The listing builds one solid part. Answer for the finished solid, in the listing's coordinates (mm). A direction names the side the tool comes from. Coordinates: 2 decimals unless noted, no trailing zeros. Order: outer loops, then holes, each group sorted by start corner. A loop starts at its lowest first (then second) coordinate and runs counter-clockwise, first axis right, second up. Notation, with made-up numbers: (12, -11) - (29, -11) arc R22 ccw to (29, 0) - close; hole circle Ø10 at (3, 50.5). An arc over 180 degrees is marked (long way). Use a Markdown table: item, result. Add a question column.
Item 1: Find the intervals of material crossed by line 1 along Z through (x, y) = (78.5, 0); line 2 along X through (y, z) = (3, 3.75); line 3 along X through (y, z) = (1.25, -3.5), in increasing order.
Item 2: The mould has two halves that part along X. Classify faces 6 (the cylindrical face through (129, -0.1, -2.9)), 7 (the flat face through (5.5, 0, -2)), 8 (the cylindrical face through (3.22, -3.75, 0.02)): released by +X, released by -X, zero draft, split by the parting line, or undercut.
Item 3: Flat-ended cylindrical pins translate along their axes: P1, Ø1, axis at x = 24.5, z = 0, coming from the -Y side; P2, Ø0.6, axis at x = 120, y = 0, coming from the +Z side; P3, Ø0.8, axis at x = 122, z = 2.5, coming from the -Y side; P4, Ø3, axis at y = -0.5, z = 0, coming from the -X side. Find the tip coordinate at first contact, or state that the pin passes through.
Item 4: The part is cut by section B-B, the plane x = 17. Give the vertices of the cut face in (y, z), then the cut area to 3 significant figures.
Item 5: For faces 1 (the flat face through (7, -4, -1)), 2 (the flat face through (3, 0, -1.25)), 3 (the flat face through (3, 0, 1.25)), 4 (the flat face through (122, 0, 1.8)), 5 (the cylindrical face through (3.22, 3.75, -0.02)), determine the directions among +Z, -Z, +X, -X, +Y, -Y from which every point of the face is accessible in a straight line to the end or side of a thin tool.
Item 6: The part is cut by section A-A, the plane z = 0. Give the vertices of the cut face in (x, y), then the cut area to 3 significant figures.
from build123d import *

# Parameters (mm, degrees)
F2_SIZE  = 1
F4_DEPTH = 5.5
F7_DEPTH = 1.2


with BuildPart() as f1:
    # F0 (on Front) → F1 (revolve)
    with BuildSketch(Plane.XZ):
        Polygon((0, 3.75), (0, 0), (130, 0), (130, 3), (129.3, 3), (129.3, 2.9), (128.7, 2.9), (128.7, 3), (115, 3), (115, 3.75), (7, 3.75), (7, 5), (5.5, 5), (5.5, 3.75), align=None)
    revolve(axis=Axis((81.1427264533, 0, 0), (1, 0, 0)))

    # F2
    f2_edges = [f1.edges().sort_by_distance(p)[0] for p in [
        (0, 0, -3.75),
    ]]
    chamfer(f2_edges, length=F2_SIZE)

    # F3 (on face) → F4 (cut, through all)
    with BuildSketch(Plane(origin=(0, 0, 0), x_dir=(0, -1, 0), z_dir=(-1, 0, 0))):
        with BuildLine():
            Line((2.4494897428, 1.25), (3.5355339059, 1.25))
            ThreePointArc((3.5355339059, 1.25), (0, 3.75), (-3.5355339059, 1.25))
            Line((-3.5355339059, 1.25), (-2.4494897428, 1.25))
            ThreePointArc((-2.4494897428, 1.25), (0, 2.75), (2.4494897428, 1.25))
        make_face()
        with BuildLine():
            ThreePointArc((-3.5355339059, -1.25), (0, -3.75), (3.5355339059, -1.25))
            Line((3.5355339059, -1.25), (2.4494897428, -1.25))
            ThreePointArc((2.4494897428, -1.25), (0, -2.75), (-2.4494897428, -1.25))
            Line((-2.4494897428, -1.25), (-3.5355339059, -1.25))
        make_face()
        with BuildLine():
            Line((-2.4494897428, 1.25), (2.4494897428, 1.25))
            ThreePointArc((2.4494897428, 1.25), (0, 2.75), (-2.4494897428, 1.25))
        make_face()
        with BuildLine():
            ThreePointArc((-2.4494897428, -1.25), (0, -2.75), (2.4494897428, -1.25))
            Line((2.4494897428, -1.25), (-2.4494897428, -1.25))
        make_face()
    extrude(amount=-F4_DEPTH, mode=Mode.SUBTRACT)

    # F6 (on offset) → F7 (cut, through all)
    with BuildSketch(Plane.XY.offset(1.8)):
        with BuildLine():
            ThreePointArc((125, -1), (126, 0), (125, 1))
            Line((125, 1), (119, 1))
            ThreePointArc((119, 1), (118, 0), (119, -1))
            Line((119, -1), (125, -1))
        make_face()
    extrude(amount=F7_DEPTH, mode=Mode.SUBTRACT)


solid = f1.part
Solution:
| question | item | result |
|---|---|---|
| 1 | line 1 | z = -3.75 to 3.75 |
| 1 | line 2 | x = 5.5 to 7 |
| 1 | line 3 | x = 5.5 to 115 |
| 2 | face 6 | undercut |
| 2 | face 7 | released by -X |
| 2 | face 8 | zero draft |
| 3 | P1 | stops at y = -3.75 |
| 3 | P2 | stops at z = 1.8 |
| 3 | P3 | stops at y = -2.14 |
| 3 | P4 | stops at x = 0 |
| 4 | outline | circle Ø7.5 at (0, 0) |
| 4 | area | 44.2 mm2 |
| 5 | face 1 | +X |
| 5 | face 2 | -Z, -X, +Y, -Y |
| 5 | face 3 | +Z, -X, +Y, -Y |
| 5 | face 4 | +Z |
| 5 | face 5 | -X, +Y |
| 6 | outline | (0, -2.75) - (1, -3.75) - (5.5, -3.75) - (5.5, -5) - (7, -5) - (7, -3.75) - (115, -3.75) - (115, -3) - (128.7, -3) - (128.7, -2.9) - (129.3, -2.9) - (129.3, -3) - (130, -3) - (130, 3) - (129.3, 3) - (129.3, 2.9) - (128.7, 2.9) - (128.7, 3) - (115, 3) - (115, 3.75) - (7, 3.75) - (7, 5) - (5.5, 5) - (5.5, 3.75) - (1, 3.75) - (0, 2.75) - close |
| 6 | area | 955 mm2 |
